from build123d import *

# Parameters (mm, degrees)
BOSS_EXTRUDE3_DEPTH = 2
SKETCH5_R           = 1.5
CUT_EXTRUDE1_DEPTH  = 2
SKETCH7_R           = 12
BOSS_EXTRUDE4_DEPTH = 6
CUT_EXTRUDE2_DEPTH  = 4
CUT_EXTRUDE3_REACH  = 321.177
SKETCH9_R           = 4


with BuildPart() as part:
    # Sketch2 → Boss-Extrude3 (new body)
    with BuildSketch(Plane(origin=(0, -145, 0), x_dir=(1, 0, 0), z_dir=(0, 1, 0))):
        with BuildLine():
            Line((266.76742756, -73.602742484), (266.76742756, -72.760276474))
            ThreePointArc((266.76742756, -72.760276474), (295.4188355, -56.546474798), (306.76742756, -25.643400517))
            Line((306.76742756, -25.643400517), (306.76742756, 17.897133595))
            ThreePointArc((306.76742756, 17.897133595), (295.4188355, 48.800207875), (266.76742756, 65.014009552))
            Line((266.76742756, 65.014009552), (266.76742756, 65.935160893))
            add(Edge.make_bspline(
                [(266.76742756, 65.935160893), (259.107155635, 65.341277023), (243.742271939, 64.387770992), (220.806823342, 63.7720731), (197.927488127, 64.011220421), (175.127118785, 65.165170469), (152.40787224, 67.285858288), (129.776603883, 70.444148029), (110.989691022, 74.011185897), (96.0146349, 77.459243676), (88.529196958, 79.398823116), (84.805077121, 80.412721287)],
                knots=[0.001455315, 0.001455315, 0.001455315, 0.001455315, 0.126054107, 0.2506529, 0.375251692, 0.499850484, 0.624449276, 0.749048068, 0.87364686, 0.935946256, 0.998245653, 0.998245653, 0.998245653, 0.998245653], degree=3))
            Line((84.805077121, 80.412721287), (84.805077121, -88.045510644))
            add(Edge.make_bspline(
                [(84.805077121, -88.045510644), (88.529310634, -87.032335524), (96.014951065, -85.094214441), (110.990402818, -81.649056168), (129.777732342, -78.085640943), (152.409330828, -74.931693387), (175.128665838, -72.815352211), (197.928863022, -71.6657552), (220.807845871, -71.43096305), (243.742803934, -72.051009048), (259.107355476, -73.007418463), (266.76742756, -73.602742484)],
                knots=[0.001754687, 0.001754687, 0.001754687, 0.001754687, 0.064054081, 0.126353476, 0.250952265, 0.375551054, 0.500149843, 0.624748632, 0.749347421, 0.873946211, 0.998545, 0.998545, 0.998545, 0.998545], degree=3))
        make_face()
    extrude(amount=BOSS_EXTRUDE3_DEPTH)

    # Sketch5 → Cut-Extrude1 (cut)
    with BuildSketch(Plane.XZ.offset(145)):
        with Locations(Location((241.293747278, 70.518625741, 0), (0, 0, 270))):
            Circle(SKETCH5_R)
        with Locations(Location((133.692207926, 75.539122499, 0), (0, 0, 270))):
            Circle(SKETCH5_R)
        with Locations(Location((133.692207926, -67.792864213, 0), (0, 0, 270))):
            Circle(SKETCH5_R)
        with Locations(Location((241.293747278, -62.772367455, 0), (0, 0, 270))):
            Circle(SKETCH5_R)
    extrude(amount=-CUT_EXTRUDE1_DEPTH, mode=Mode.SUBTRACT)

    # Sketch7 → Boss-Extrude4 (add)
    with BuildSketch(Plane.XZ.offset(145)):
        with Locations(Location((216.15176331, 3.918032565, 0), (0, 0, 270))):
            Circle(SKETCH7_R)
    extrude(amount=-BOSS_EXTRUDE4_DEPTH)

    # Sketch8 → Cut-Extrude2 (cut)
    with BuildSketch(Plane.XZ.offset(145)):
        Polygon((219.337574148, -2.87784432), (223.630070752, 3.279087239), (220.444259915, 10.074964125), (212.965952472, 10.71390945), (208.673455868, 4.556977891), (211.859266705, -2.238898995), align=None)
    extrude(amount=-CUT_EXTRUDE2_DEPTH, mode=Mode.SUBTRACT)

    # Sketch9 → Cut-Extrude3 (cut, up to next)
    with BuildSketch(Plane.XZ.offset(141), mode=Mode.PRIVATE) as cut_extrude3_sk1:
        with Locations(Location((216.15176331, 3.918032565, 0), (0, 0, 270))):
            Circle(SKETCH9_R)
    cut_extrude3_tool1 = extrude(cut_extrude3_sk1.sketch, amount=-CUT_EXTRUDE3_REACH, mode=Mode.PRIVATE) & part.part
    add(cut_extrude3_tool1.solids().sort_by_distance((216.151763, -141, 3.918033))[0], mode=Mode.SUBTRACT)


solid = part.part
Input: part model. Units: mm. Frame: model coordinates. A direction names the side the tool comes from. Give positions to 0.01 mm unless a question says otherwise; leave off trailing zeros. Write each loop counter-clockwise with the first axis right and the second up, starting at its lowest first coordinate (ties: lowest second). Pieces come first, ordered by that corner, then holes. Notation, with made-up numbers: M 67.5,43 L 112.5,43 A29 ccw 112.5,63 Z; hole C -8,30.25 d1. An arc over 180 degrees is marked long. Write item = value, one per line. Start each with the question number.
1) Draft query along X for faces 1 (the flat face through (213, -141, 1)), 2 (the flat face through (219, -139, 7)), 3 (the flat face through (221.454, -143.028, 0.158)), 4 (the cylindrical face through (295.72, -144.01, -48.44)). Return one class per face: +X half, -X half, draft (parallel to the pull), parting line (faces both ways), or undercut.
2) Material intervals for line 1 along Y through (x, z) = (287.5, 36); line 2 along X through (y, z) = (-143.25, -2); line 3 along X through (y, z) = (-142, 2.5), sorted ascending. Write a range as [from, to].
3) First-contact query: pin 1 Ø10 at (x, z) = (154.5, 53.5) entering from +Y; pin 2 Ø0.7 at (y, z) = (-144.5, -65.5) entering from +X. Flat tips, straight axial feed; report the tip coordinate or a pass-through.
4) Cut plane B-B on x = 275.5. Return the cut outline in (y, z).
5) Cut plane C-C on y = -144. Count the separate pieces of the cut face and the enclosed holes in it, then the cut area to 3 significant figures.
6) Reachability of faces 5 (the flat face through (210.85, -143.03, 7.68)), 6 (the cylindrical face through (212.25, -140.01, 4.79)), 7 (the cylindrical face through (226.27, -141.03, -2.53)) from +Z, -Z, +X, -X, +Y, -Y: full face, straight path, thin tool, end or side. Return the list, or none.
7) Cut plane A-A on z = -54.5. Return the cut outline in (x, y).
Solved:
q1.face_1 = undercut
q1.face_2 = draft
q1.face_3 = undercut
q1.face_4 = +X half
q2.line_1 = [-145, -143]
q2.line_2 = [84.81, 211.75], [219.95, 306.77]
q2.line_3 = [204.24, 209.64], [223.09, 228.07]
q3.pin_1 = -143
q3.pin_2 = 266.77
q4.outline = M -145,-62.71 L -143,-62.71 L -143,70.46 L -145,70.46 Z
q5.separate_pieces = 1
q5.enclosed_holes = 5
q5.area = 30,500 mm2
q6.face_5 = -Y
q6.face_6 = +Y, -Y
q6.face_7 = +Y
q7.outline = M 84.81,-145 L 289.68,-145 L 289.68,-143 L 84.81,-143 Z
